Design review of the part built by this model. Coordinates are the model's own, in mm. A direction names the side the tool comes from. Give positions to 0.01 mm unless a question says otherwise; leave off trailing zeros. Write each loop counter-clockwise with the first axis right and the second up, starting at its lowest first coordinate (ties: lowest second). Pieces come first, ordered by that corner, then holes. Notation, with made-up numbers: (74, 29.25) -> (124, 29.25) arc R4 cw to (124, 35.25) -> close; hole circle Ø4 at (88.25, 89). An arc over 180 degrees is marked (long way). Answer as a JSON object with one key per item and string values.
```python
from build123d import *

# Parameters (mm, degrees)
F0_R          = 18.5884572681
F1_DEPTH      = 30
F2_R          = 2
F3_DEPTH      = 5.0894572681
F3_DEPTH_BACK = 32.0894572681


# Not quite as in the source:
# - a feature names something its author has since deleted; it is built from what else it names


with BuildPart() as f1:
    # F0 (on Top) → F1 (new body)
    with BuildSketch(Plane.XY):
        Circle(F0_R)
        Polygon((0, 15.5884572681), (13.5, 7.7942286341), (13.5, -7.7942286341), (0, -15.5884572681), (-13.5, -7.7942286341), (-13.5, 7.7942286341), align=None, mode=Mode.SUBTRACT)
    extrude(amount=F1_DEPTH)

    # F2 (on face) → F3 (cut, two sides)
    with BuildSketch(Plane.YZ.offset(-13.5)) as f3_sk:
        with Locations((0, 22.5)):
            Circle(F2_R)
    extrude(amount=-F3_DEPTH, mode=Mode.SUBTRACT)
    extrude(f3_sk.sketch, amount=F3_DEPTH_BACK, mode=Mode.SUBTRACT)


solid = f1.part
```
(1) We need section D-D, the plane y = -11.5. State the section outline as (x, z) points.
Here are the results:
{"outline": "(-14.6, 0) -> (-7.08, 0) -> (-7.08, 30) -> (-14.6, 30) -> close; (7.08, 0) -> (14.6, 0) -> (14.6, 30) -> (7.08, 30) -> close"}
(2) We need section C-C, the plane z = 10.5. State the section outline as (x, y) points.
Here are the results:
{"outline": "circle Ø37.18 at (0, 0); hole (-13.5, -7.79) -> (0, -15.59) -> (13.5, -7.79) -> (13.5, 7.79) -> (0, 15.59) -> (-13.5, 7.79) -> close"}
(3) Clearance check with flat-ended pins moving along their axes: pin 1 (1.5 mm diameter, centred on y = 0.5, z = 23, fed in from +X); pin 2 (12 mm diameter, centred on y = 14.5, z = 22, fed in from -X); pin 3 (1.5 mm diameter, centred on y = 1.5, z = 4.5, fed in from -X); pin 4 (10 mm diameter, centred on x = 5.5, y = 8.5, fed in from +Z). State where each tip first meets the part, or that it passes through.
Here are the results:
{"pin 1": "passes through", "pin 2": "stops at x = -16.53", "pin 3": "stops at x = -18.57", "pin 4": "stops at z = 30"}
(4) We need section A-A, the plane x = 6.5. State the section outline as (y, z) points.
Here are the results:
{"outline": "(-17.41, 0) -> (-11.84, 0) -> (-11.84, 30) -> (-17.41, 30) -> close; (11.84, 0) -> (17.41, 0) -> (17.41, 30) -> (11.84, 30) -> close"}
(5) The part is to be moulded in two halves that separate along Z. For faces 1 (the flat face through (14, -1, 0)), 2 (the flat face through (14, -1, 30)), 3 (the flat face through (-6.84, 11.64, 14.79)), 4 (the cylindrical face through (16.009, 0.923, 20.726)), say which applies: +Z half, -Z half, draft (parallel to the pull), parting line (faces both ways), or undercut.
Here are the results:
{"face 1": "-Z half", "face 2": "+Z half", "face 3": "draft", "face 4": "undercut"}
(6) For faces 5 (the flat face through (6.84, -11.64, 14.79)), 6 (the cylindrical face through (-16.009, 0.923, 20.726)), list the 3-axis set-ups (+Z, -Z, +X, -X, +Y, -Y) from which the entire face can be reached by the end or side of a thin tool; tool diameter is ignored.
Here are the results:
{"face 5": "+Z, -Z", "face 6": "+X, -X"}
(7) For line 1 along Z through (x, y) = (16.85, 0); line 2 along X through (y, z) = (-0.5, 14); line 3 along Y through (x, z) = (-2, 18.5), list the stretches that pass through material, from the lowest coordinate up.
Here are the results:
{"line 1": "z = 0 to 20.5, 24.5 to 30", "line 2": "x = -18.58 to -13.5, 13.5 to 18.58", "line 3": "y = -18.48 to -14.43, 14.43 to 18.48"}
(8) We need section B-B, the plane y = 0. State the section outline as (x, z) points.
Here are the results:
{"outline": "(-18.59, 0) -> (-13.5, 0) -> (-13.5, 20.5) -> (-18.59, 20.5) -> close; (-18.59, 24.5) -> (-13.5, 24.5) -> (-13.5, 30) -> (-18.59, 30) -> close; (13.5, 0) -> (18.59, 0) -> (18.59, 20.5) -> (13.5, 20.5) -> close; (13.5, 24.5) -> (18.59, 24.5) -> (18.59, 30) -> (13.5, 30) -> close"}
